Could you check a few things on this model? Use its own coordinates, in mm. Face numbers are marked on the shaded views. A direction names the side the tool comes from. Round coordinates to 2 decimals unless told otherwise and drop trailing zeros. Write each loop counter-clockwise with the first axis right and the second up, starting at its lowest first coordinate (ties: lowest second). Pieces come first, ordered by that corner, then holes. Notation, with made-up numbers: (56, 79.5) -> (86, 79.5) arc R23 cw to (86, 92.5) -> close; hole circle Ø9 at (0, 64.5). An arc over 180 degrees is marked (long way). Answer as CSV lines item,"result". Start each with the question number.
Q1. Imagine slicing it at D-D on z = -3. Please give me the cut outline in (x, y), and give its area (3 significant figures).
Q2. Imagine slicing it at C-C on z = -21.75. Please give me the cut outline in (x, y), and give its area (3 significant figures).
Q3. For the marked faces 1, 2 and 3, which set-ups out of +Z, -Z, +X, -X, +Y, -Y let a thin tool reach every point of the face, with its end or its side?
Q4. Imagine slicing it at A-A on y = 0. Please give me the cut outline in (x, z).
Q5. If I drill on line 1 (Z direction, x = 3.5, y = -7); line 2 (X direction, y = 0.25, z = -9.5); line 3 (Z direction, x = -3.25, y = -7.5), over which ranges is the centre line in solid material (lowest first)? Write a range as [from, to].
Q6. Imagine slicing it at B-B on x = 0. Please give me the cut outline in (y, z), and give its area (3 significant figures).
Q7. Will these pins go through, and if not, where does the flat tip stop? pin 1 Ø1 at (x, z) = (0.5, 2.5) entering from -Y; pin 2 Ø1 at (x, z) = (-0.5, -22) entering from -Y; pin 3 Ø4 at (y, z) = (-1, -3.5) entering from -X.
from build123d import *

# Parameters (mm, degrees)
SKETCH_1_R          = 11.25
EXTRUDE_1_DEPTH     = 4
CHAMFER_1_SIZE      = 3
SKETCH_2_W          = 6
SKETCH_2_H          = 3
CUT_EXTRUDE_1_DEPTH = 2
EXTRUDE_2_DEPTH     = 18
SKETCH_4_R          = 6.25
EXTRUDE_3_DEPTH     = 7.5


with BuildPart() as part:
    # 草图1 → 拉伸1 (new body)
    with BuildSketch(Plane.XY):
        Circle(SKETCH_1_R)
    extrude(amount=EXTRUDE_1_DEPTH)

    # 倒角1
    chamfer_1_edges = [part.edges().sort_by_distance(p)[0] for p in [
        (-11.25, 0, 4),
    ]]
    chamfer(chamfer_1_edges, length=CHAMFER_1_SIZE)

    # 草图2 → 切除-拉伸1 (cut)
    with BuildSketch(Plane.XY.offset(4)):
        Rectangle(SKETCH_2_W, SKETCH_2_H)
    extrude(amount=-CUT_EXTRUDE_1_DEPTH, mode=Mode.SUBTRACT)

    # 草图3 → 拉伸2 (add)
    with BuildSketch(Plane(origin=(0, 0, 0), x_dir=(-1, 0, 0), z_dir=(0, 0, -1))):
        with BuildLine():
            Line((-7.5, 2.783882181), (-7.5, -2.783882181))
            ThreePointArc((-7.5, -2.783882181), (0, -8), (7.5, -2.783882181))
            Line((7.5, -2.783882181), (7.5, 2.783882181))
            ThreePointArc((7.5, 2.783882181), (0, 8), (-7.5, 2.783882181))
        make_face()
    extrude(amount=EXTRUDE_2_DEPTH)

    # 草图4 → 拉伸3 (add)
    with BuildSketch(Plane(origin=(0, 0, -18), x_dir=(-1, 0, 0), z_dir=(0, 0, -1))):
        with Locations(Location((0, 0, 0), (0, 0, 180))):
            Circle(SKETCH_4_R)
    extrude(amount=EXTRUDE_3_DEPTH)


solid = part.part
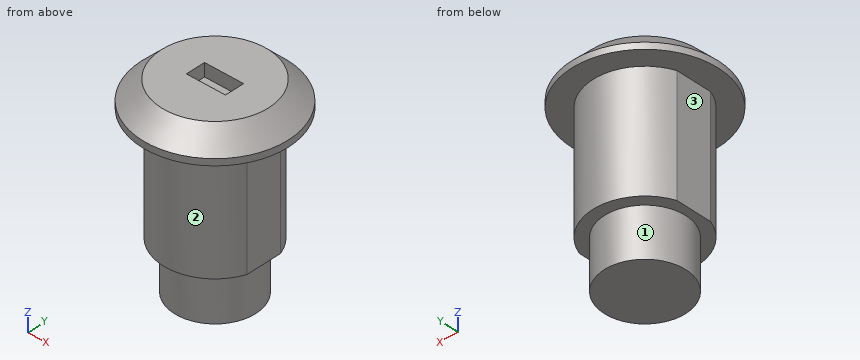
Checks:
1,outline,"(-7.5, -2.78) arc R8 ccw to (7.5, -2.78) -> (7.5, 2.78) arc R8 ccw to (-7.5, 2.78) -> close"
1,area,"197 mm^2"
2,outline,"circle Ø12.5 at (0, 0)"
2,area,"123 mm^2"
3,face 1,"-Z"
3,face 2,"-Z, -Y"
3,face 3,"-Z, -X, +Y, -Y"
4,outline,"(-11.25, 0) -> (-7.5, 0) -> (-7.5, -18) -> (-6.25, -18) -> (-6.25, -25.5) -> (6.25, -25.5) -> (6.25, -18) -> (7.5, -18) -> (7.5, 0) -> (11.25, 0) -> (11.25, 1) -> (8.25, 4) -> (3, 4) -> (3, 2) -> (-3, 2) -> (-3, 4) -> (-8.25, 4) -> (-11.25, 1) -> close"
5,line 1,"[-18, 4]"
5,line 2,"[-7.5, 7.5]"
5,line 3,"[0, 4]"
6,outline,"(-11.25, 0) -> (-8, 0) -> (-8, -18) -> (-6.25, -18) -> (-6.25, -25.5) -> (6.25, -25.5) -> (6.25, -18) -> (8, -18) -> (8, 0) -> (11.25, 0) -> (11.25, 1) -> (8.25, 4) -> (1.5, 4) -> (1.5, 2) -> (-1.5, 2) -> (-1.5, 4) -> (-8.25, 4) -> (-11.25, 1) -> close"
6,area,"457 mm^2"
7,pin 1,"y = -10.24"
7,pin 2,"y = -6.25"
7,pin 3,"x = -7.5"
